Input: part model. Units: mm. Frame: model coordinates. Round coordinates to 2 decimals unless told otherwise and drop trailing zeros. Loops run counter-clockwise (first coordinate to the right, second up) from the corner with the lowest first, then second, coordinate; pieces in that order, holes last. Notation, with made-up numbers: (-17, 70) - (12, 70) arc R29 ccw to (12, 96) - close; hole circle Ø6 at (-26, 40). An arc over 180 degrees is marked (long way). Use CSV: the item, a comma, the result in double quotes. Start each with the question number.
1. Cut plane C-C (y = 0.3). Give the number of separate pieces and of enclosed holes in the cut face, and give its area (3 significant figures).
2. Pin query (flat end, axial travel): P1, Ø0.5, axis at x = 11.5, y = 0.5, coming from the -Z side. Return the tip coordinate at first contact, or that it passes through.
3. Material intervals for probe 1 along Z at (x, y) = (16.25, 0.85); probe 2 along X at (y, z) = (0.1, -12); probe 3 along X at (y, z) = (0.9, -9.5), sorted ascending. Write a range as from..to.
4. Cut plane B-B (z = 14). Return loops of the section in (x, y).
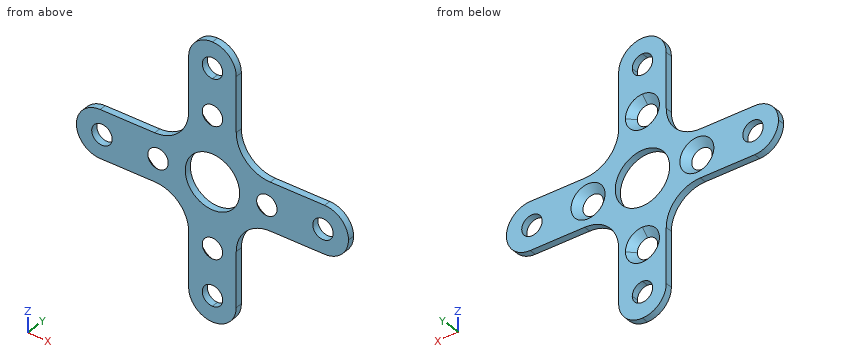
```python
from build123d import *

# Parameters (mm, degrees)
SKETCH1_W           = 3.5
SKETCH1_H           = 3.5
BOSS_EXTRUDE1_DEPTH = 1
FILLET1_R           = 5
FILLET2_R           = 3.5
CUT_EXTRUDE1_REACH  = 30.302
SKETCH2_R           = 4
CHAMFER1_SIZE       = 1


with BuildPart() as part:
    # Sketch1 → Boss-Extrude1 (new body)
    with BuildSketch(Plane(origin=(0, 0, 0), x_dir=(1, 0, 0), z_dir=(0, 1, 0))):
        with BuildLine():
            Line((-6.5, 0), (-3.5, 0))
            Line((-3.5, 0), (-3.5, 3.5))
            Line((-3.5, 3.5), (-20, 3.5))
            Line((-20, 3.5), (-20, 0))
            Line((-20, 0), (-17.75, 0))
            ThreePointArc((-17.75, 0), (-16.25, 1.5), (-14.75, 0))
            Line((-14.75, 0), (-9.5, 0))
            ThreePointArc((-9.5, 0), (-8, 1.5), (-6.5, 0))
        make_face()
        with BuildLine():
            Line((-20, -3.5), (-3.5, -3.5))
            Line((-3.5, -3.5), (-3.5, 0))
            Line((-3.5, 0), (-6.5, 0))
            ThreePointArc((-6.5, 0), (-8, -1.5), (-9.5, 0))
            Line((-9.5, 0), (-14.75, 0))
            ThreePointArc((-14.75, 0), (-16.25, -1.5), (-17.75, 0))
            Line((-17.75, 0), (-20, 0))
            Line((-20, 0), (-20, -3.5))
        make_face()
        with BuildLine():
            Line((-3.5, 20), (-3.5, 3.5))
            Line((-3.5, 3.5), (0, 3.5))
            Line((0, 3.5), (0, 8))
            ThreePointArc((0, 8), (-1.5, 9.5), (0, 11))
            Line((0, 11), (0, 14.75))
            ThreePointArc((0, 14.75), (-1.5, 16.25), (0, 17.75))
            Line((0, 17.75), (0, 20))
            Line((0, 20), (-3.5, 20))
        make_face()
        with BuildLine():
            Line((0, 3.5), (3.5, 3.5))
            Line((3.5, 3.5), (3.5, 20))
            Line((3.5, 20), (0, 20))
            Line((0, 20), (0, 17.75))
            ThreePointArc((0, 17.75), (1.060660172, 17.310660172), (1.5, 16.25))
            ThreePointArc((1.5, 16.25), (1.060660172, 15.189339828), (0, 14.75))
            Line((0, 14.75), (0, 11))
            ThreePointArc((0, 11), (1.060660172, 10.560660172), (1.5, 9.5))
            ThreePointArc((1.5, 9.5), (1.060660172, 8.439339828), (0, 8))
            Line((0, 8), (0, 3.5))
        make_face()
        with BuildLine():
            Line((3.5, 3.5), (3.5, 0))
            Line((3.5, 0), (6.5, 0))
            ThreePointArc((6.5, 0), (8, 1.5), (9.5, 0))
            Line((9.5, 0), (14.75, 0))
            ThreePointArc((14.75, 0), (16.25, 1.5), (17.75, 0))
            Line((17.75, 0), (20, 0))
            Line((20, 0), (20, 3.5))
            Line((20, 3.5), (3.5, 3.5))
        make_face()
        with Locations((-1.75, 1.75)):
            Rectangle(SKETCH1_W, SKETCH1_H)
        with Locations((-1.75, -1.75)):
            Rectangle(SKETCH1_W, SKETCH1_H)
        with Locations((1.75, -1.75)):
            Rectangle(SKETCH1_W, SKETCH1_H)
        with Locations((1.75, 1.75)):
            Rectangle(SKETCH1_W, SKETCH1_H)
        with BuildLine():
            Line((-3.5, -20), (0, -20))
            Line((0, -20), (0, -17.75))
            ThreePointArc((0, -17.75), (-1.5, -16.25), (0, -14.75))
            Line((0, -14.75), (0, -11))
            ThreePointArc((0, -11), (-1.5, -9.5), (0, -8))
            Line((0, -8), (0, -3.5))
            Line((0, -3.5), (-3.5, -3.5))
            Line((-3.5, -3.5), (-3.5, -20))
        make_face()
        with BuildLine():
            Line((0, -17.75), (0, -20))
            Line((0, -20), (3.5, -20))
            Line((3.5, -20), (3.5, -3.5))
            Line((3.5, -3.5), (0, -3.5))
            Line((0, -3.5), (0, -8))
            ThreePointArc((0, -8), (1.060660172, -8.439339828), (1.5, -9.5))
            ThreePointArc((1.5, -9.5), (1.060660172, -10.560660172), (0, -11))
            Line((0, -11), (0, -14.75))
            ThreePointArc((0, -14.75), (1.060660172, -15.189339828), (1.5, -16.25))
            ThreePointArc((1.5, -16.25), (1.060660172, -17.310660172), (0, -17.75))
        make_face()
        with BuildLine():
            Line((3.5, 0), (3.5, -3.5))
            Line((3.5, -3.5), (20, -3.5))
            Line((20, -3.5), (20, 0))
            Line((20, 0), (17.75, 0))
            ThreePointArc((17.75, 0), (16.25, -1.5), (14.75, 0))
            Line((14.75, 0), (9.5, 0))
            ThreePointArc((9.5, 0), (8, -1.5), (6.5, 0))
            Line((6.5, 0), (3.5, 0))
        make_face()
    extrude(amount=BOSS_EXTRUDE1_DEPTH)

    # Fillet1
    fillet1_edges = [part.edges().sort_by_distance(p)[0] for p in [
        (-3.5, 0.5, -3.5),
        (3.5, 0.5, -3.5),
        (3.5, 0.5, 3.5),
        (-3.5, 0.5, 3.5),
    ]]
    fillet(fillet1_edges, radius=FILLET1_R)

    # Fillet2
    fillet2_edges = [part.edges().sort_by_distance(p)[0] for p in [
        (20, 0.5, 3.5),
        (20, 0.5, -3.5),
        (3.5, 0.5, -20),
        (-3.5, 0.5, -20),
        (-20, 0.5, -3.5),
        (-20, 0.5, 3.5),
        (3.5, 0.5, 20),
        (-3.5, 0.5, 20),
    ]]
    fillet(fillet2_edges, radius=FILLET2_R - 0.0001)  # a hair under: the kernel refuses the full size

    # Sketch2 → Cut-Extrude1 (cut, up to next)
    with BuildSketch(Plane(origin=(0, 1, 0), x_dir=(1, 0, 0), z_dir=(0, 1, 0)), mode=Mode.PRIVATE) as cut_extrude1_sk1:
        with Locations(Location((0, 0, 0), (0, 0, 270))):
            Circle(SKETCH2_R)
    cut_extrude1_tool1 = extrude(cut_extrude1_sk1.sketch, amount=-CUT_EXTRUDE1_REACH, mode=Mode.PRIVATE) & part.part
    add(cut_extrude1_tool1.solids().sort_by_distance((0, 1, 0))[0], mode=Mode.SUBTRACT)

    # Chamfer1
    chamfer1_edges = [part.edges().sort_by_distance(p)[0] for p in [
        (0, 1, 11),
        (6.5, 1, 0),
        (-6.5, 1, 0),
        (0, 1, -11),
    ]]
    chamfer(chamfer1_edges, length=CHAMFER1_SIZE - 0.0001)  # a hair under: the kernel refuses the full size


solid = part.part
```
Established:
1,separate pieces,"1"
1,enclosed holes,"9"
1,area,"392 mm2"
2,P1,"stops at z = -3.5"
3,probe 1,"z = -3.5..-1.5, 1.5..3.5"
3,probe 2,"x = -3.5..3.5"
3,probe 3,"x = -3.5..-2.4, 2.4..3.5"
4,outline,"(-3.5, 0) - (3.5, 0) - (3.5, 1) - (-3.5, 1) - close"
